Check sheet for the modelled part. Datum: model origin and axes. Units: mm. Round coordinates to 2 decimals unless told otherwise and drop trailing zeros. Loops run counter-clockwise (first coordinate to the right, second up) from the corner with the lowest first, then second, coordinate; pieces in that order, holes last. Notation, with made-up numbers: (4.25, 44.25) - (25.25, 44.25) arc R29 ccw to (25.25, 68.25) - close; hole circle Ø2 at (60.25, -14.5). An arc over 180 degrees is marked (long way). Return JSON: item names as keys, results as strings.
from build123d import *

# Parameters (mm, degrees)
F0_W          = 152.138144
F0_H          = 55.172988
F1_DEPTH      = 35.56
F1_DEPTH_BACK = 35.56
F2_R          = 32.536821
F3_DEPTH      = 74.65833
F4_R          = 16.891658
F5_DEPTH      = 60.75289
F7_DEPTH      = 58.39537


with BuildPart() as f1:
    # F0 (on Front) → F1 (new body, two sides)
    with BuildSketch(Plane.XZ) as f1_sk:
        Rectangle(F0_W, F0_H)
    extrude(amount=F1_DEPTH)
    extrude(f1_sk.sketch, amount=-F1_DEPTH_BACK)

    # F2 (on face) → F3 (cut)
    with BuildSketch(Plane.XZ.offset(35.56)):
        with Locations((37.392992, 14.286671)):
            Circle(F2_R)
    extrude(amount=-F3_DEPTH, mode=Mode.SUBTRACT)

    # F4 (on face) → F5 (cut)
    with BuildSketch(Plane.XY.offset(27.586494)):
        with Locations((-36.354639, 0)):
            Circle(F4_R)
    extrude(amount=-F5_DEPTH, mode=Mode.SUBTRACT)

    # F6 (on face) → F7 (cut)
    with BuildSketch(Plane.XY.offset(27.586494)):
        Polygon((-76.069072, -13.85648), (-76.069072, -35.56), (-56.617878, -35.56), align=None)
        Polygon((-76.069072, 13.85648), (-56.617878, 35.56), (-76.069072, 35.56), align=None)
    extrude(amount=-F7_DEPTH, mode=Mode.SUBTRACT)


solid = f1.part
Q1. Draft check along Z on faces 1 (the face through (-76.069, 0, 0)), 2 (the face through (72, 0, 27.586)), 3 (the face through (36.486, -0.498, -18.237)). Enter one of: released by +Z, released by -Z, zero draft, split by the parting line, or undercut.
Answer key:
{"face 1": "zero draft", "face 2": "released by +Z", "face 3": "undercut"}
Q2. Scan lines: probe 1 along X at (y, z) = (10.5, -7); probe 2 along X at (y, z) = (3.5, 5.5); probe 3 along X at (y, z) = (1, -20). Record each from-to range of solid material in increasing order. Write a range as [from, to].
Answer key:
{"probe 1": "x = [-76.07, -49.59], [-23.12, 12.79], [62, 76.07]", "probe 2": "x = [-76.07, -52.88], [-19.83, 6.07], [68.72, 76.07]", "probe 3": "x = [-76.07, -53.22], [-19.49, 76.07]"}
Q3. Sectioned sample at C-C (x = -46). Enter the section's corners in (y, z), plus the area to 3 significant figures.
Answer key:
{"outline": "(-35.56, -27.59) - (-13.87, -27.59) - (-13.87, 27.59) - (-35.56, 27.59) - close; (13.87, -27.59) - (35.56, -27.59) - (35.56, 27.59) - (13.87, 27.59) - close", "area": "2,390 mm²"}
Q4. Sectioned sample at B-B (z = 8). Enter the section's corners in (x, y), plus the area to 3 significant figures.
Answer key:
{"outline": "(-76.07, -13.86) - (-56.62, -35.56) - (5.47, -35.56) - (5.47, 35.56) - (-56.62, 35.56) - (-76.07, 13.86) - close; (69.32, -35.56) - (76.07, -35.56) - (76.07, 35.56) - (69.32, 35.56) - close; hole circle Ø33.78 at (-36.35, 0)", "area": "4,960 mm²"}
Q5. Sectioned sample at D-D (z = 19.5). Enter the section's corners in (x, y).
Answer key:
{"outline": "(-76.07, -13.86) - (-56.62, -35.56) - (5.28, -35.56) - (5.28, 35.56) - (-56.62, 35.56) - (-76.07, 13.86) - close; (69.51, -35.56) - (76.07, -35.56) - (76.07, 35.56) - (69.51, 35.56) - close; hole circle Ø33.78 at (-36.35, 0)"}
Q6. Depth check by flat-ended pin: P1, Ø10, axis at x = -26.5, y = 13.5, coming from the +Z side; P2, Ø6, axis at x = -60.5, z = 2, coming from the -Y side. Enter the tip coordinate at first touch or a pass-through.
Answer key:
{"P1": "stops at z = 27.59", "P2": "stops at y = -34.58"}
Q7. Sectioned sample at A-A (y = 0). Enter the section's corners in (x, z).
Answer key:
{"outline": "(-76.07, -27.59) - (-53.25, -27.59) - (-53.25, 27.59) - (-76.07, 27.59) - close; (-19.46, -27.59) - (76.07, -27.59) - (76.07, 27.59) - (67.09, 27.59) arc R32.54 cw (long way) to (7.7, 27.59) - (-19.46, 27.59) - close"}
